Verification items for the finished model (mm, model axes). Face numbers are marked on the shaded views. A direction names the side the tool comes from. Round coordinates to 2 decimals unless told otherwise and drop trailing zeros. Order: outer loops, then holes, each group sorted by start corner. A loop starts at its lowest first (then second) coordinate and runs counter-clockwise, first axis right, second up.
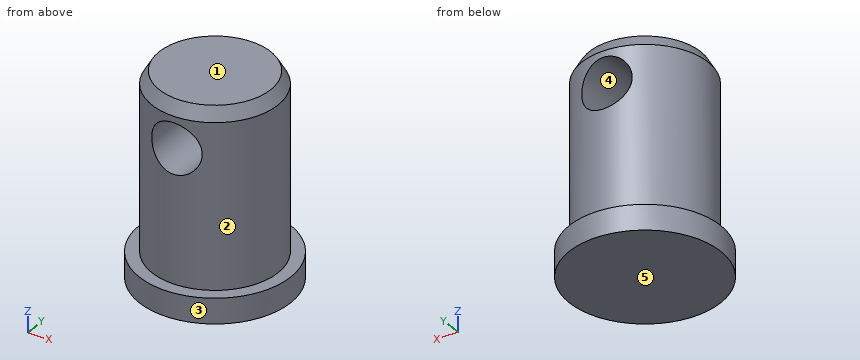
```python
from build123d import *

# Parameters (mm, degrees)
SKETCH_1_R               = 3
EXTRUDE_1_DEPTH          = 1
SKETCH_1_3_R             = 2.5
EXTRUDE_2_DEPTH          = 8
CHAMFER_1_SIZE           = 0.5
CHAMFER_1_SIZE2          = 0.288675135
CUT_EXTRUDE_1_DEPTH      = 10.055385138
CUT_EXTRUDE_1_DEPTH_BACK = 10.055385138
SKETCH_2_R               = 1


with BuildPart() as part:
    # Sketch 1 → Extrude 1 (new body)
    with BuildSketch(Plane.XY):
        Circle(SKETCH_1_R)
    extrude(amount=EXTRUDE_1_DEPTH)

    # Sketch 1_3 → Extrude 2 (add)
    with BuildSketch(Plane.XY):
        Circle(SKETCH_1_3_R)
    extrude(amount=EXTRUDE_2_DEPTH)

    # Chamfer 1
    chamfer_1_edges = [part.edges().sort_by_distance(p)[0] for p in [
        (-2.5, 0, 8),
    ]]
    chamfer_1_side = [part.faces().sort_by_distance(p)[0] for p in [
        (-2.5, 0, 4.5),
    ]]
    chamfer(chamfer_1_edges, length=CHAMFER_1_SIZE, length2=CHAMFER_1_SIZE2, reference=chamfer_1_side[0])

    # Sketch 2 → Cut-Extrude 1 (cut, two sides: drawn at the far end of the back side and taken through both)
    with BuildSketch(Plane(origin=(0, 0, 0), x_dir=(1, 0, 0), z_dir=(0, 1, 0)).offset(-CUT_EXTRUDE_1_DEPTH_BACK)):
        with Locations(Location((0, -6.25, 0), (0, 0, 270))):
            Circle(SKETCH_2_R)
    extrude(amount=CUT_EXTRUDE_1_DEPTH + CUT_EXTRUDE_1_DEPTH_BACK, mode=Mode.SUBTRACT)


solid = part.part
```
1) Sectioned sample at B-B on x = 0. Record the cut outline in (y, z).
2) Draft check along X on the marked faces 3, 4 and 5. Enter one of: released by +X, released by -X, zero draft, split by the parting line, or undercut.
3) Sectioned sample at C-C on z = 3.25. Record the cut outline in (x, y), then the cut area to 3 significant figures.
4) Sectioned sample at A-A on y = 0. Record the cut outline in (x, z).
5) Scan lines: probe 1 along Z at (x, y) = (0, 2.05); probe 2 along X at (y, z) = (0, 6.25); probe 3 along Z at (x, y) = (2.6, -1). Record each from-to range of solid material in increasing order.
6) Sectioned sample at D-D on z = 6.25. Record the cut outline in (x, y), then the cut area to 3 significant figures.
7) Go/stop test with flat-tipped pins: pin 1 Ø3 at (x, z) = (0, 6.25) entering from +Y; pin 2 Ø1 at (x, z) = (-1, 3) entering from -Y; pin 3 Ø1.5 at (x, y) = (2, -1) entering from +Z; pin 4 Ø2 at (y, z) = (1.5, 6.5) entering from -X. Record where each tip stops, or that it passes through.
8) Tool access check on the marked faces 1 and 2. Record the directions out of +Z, -Z, +X, -X, +Y, -Y that give a thin tool (end or side, any length) a straight path to the whole face; none if there is none.
Returned:
1. outline: (-3, 0) - (3, 0) - (3, 1) - (2.5, 1) - (2.5, 5.25) - (-2.5, 5.25) - (-2.5, 1) - (-3, 1) - close; (-2.5, 7.25) - (2.5, 7.25) - (2.5, 7.5) - (2.21, 8) - (-2.21, 8) - (-2.5, 7.5) - close
2. face 3: split by the parting line
2. face 4: undercut
2. face 5: zero draft
3. outline: circle Ø5 at (0, 0)
3. area: 19.6 mm2
4. outline: (-3, 0) - (3, 0) - (3, 1) - (2.5, 1) - (2.5, 7.5) - (2.21, 8) - (-2.21, 8) - (-2.5, 7.5) - (-2.5, 1) - (-3, 1) - close; hole circle Ø2 at (0, 6.25)
5. probe 1: z = 0 to 5.25, 7.25 to 8
5. probe 2: x = -2.5 to -1, 1 to 2.5
5. probe 3: z = 0 to 1
6. outline: (-1, -2.29) - (-1, 2.29) arc R2.5 ccw to start; (1, -2.29) arc R2.5 ccw to (1, 2.29) - close
6. area: 9.91 mm2
7. pin 1: stops at y = 2.5
7. pin 2: stops at y = -2.45
7. pin 3: stops at z = 8
7. pin 4: stops at x = -2.45
8. face 1: +Z, +X, -X, +Y, -Y
8. face 2: +Z
